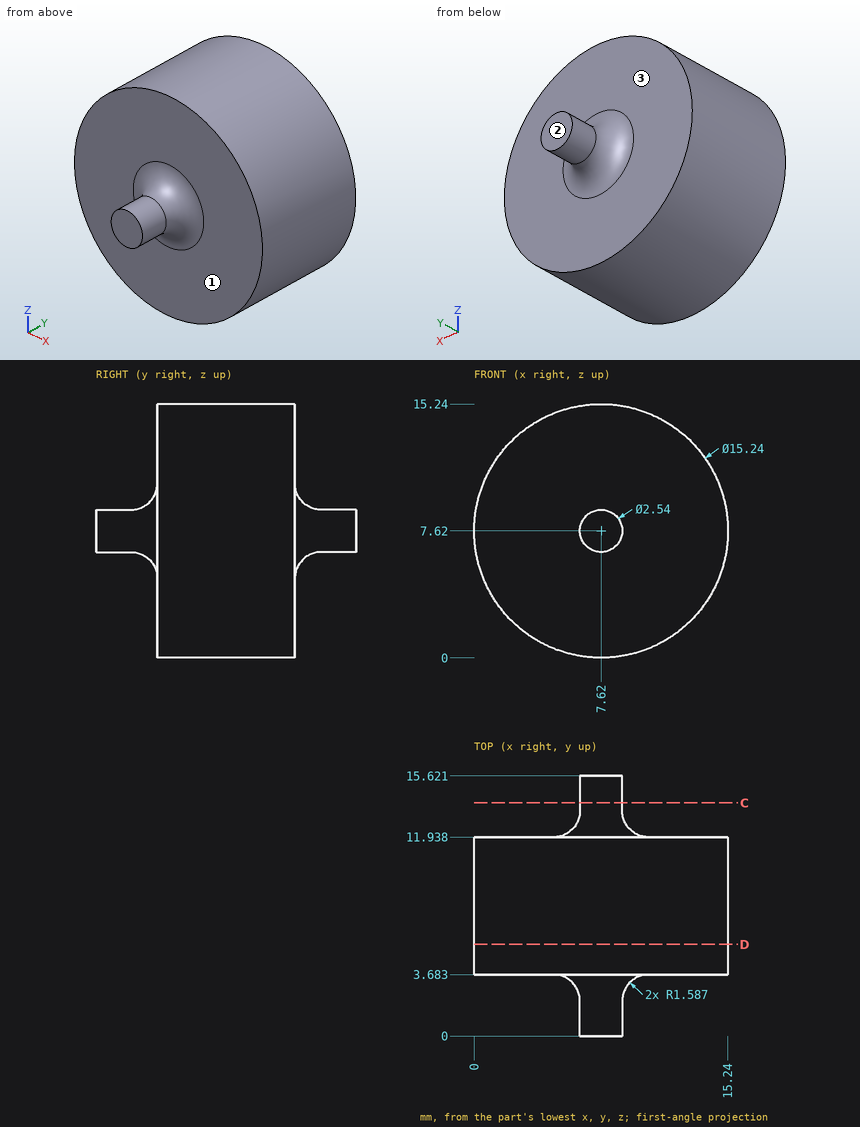
Part print with two shaded views. Sizes in mm from the minimum x, y, z corner. A direction names the side the tool comes from. Coordinates: 2 decimals unless noted, no trailing zeros. Order: outer loops, then holes, each group sorted by start corner. A loop starts at its lowest first (then second) coordinate and runs counter-clockwise, first axis right, second up.
(1) Saw through at D-D, the plane y = 5.5. Write the cut outline in (x, z).
Solution:
outline: circle Ø15.24 at (7.62, 7.62)
(2) Which spindle directions (+Z, -Z, +X, -X, +Y, -Y) get a long thin tool onto all of the face, cutting with end or side? Do the marked faces 1, 2 and 3. Say none if no direction does.
Solution:
face 1: -Y
face 2: +Z, -Z, +X, -X, +Y
face 3: +Y
(3) Drill centre lines: L1, parallel to Y at x = 14.25, z = 10; L2, parallel to Z at x = 8.75, y = 6.5 (1 decimal); L3, parallel to Z at x = 9.75, y = 7.75 (1 decimal). Where is each one in solid material? Low to high.
Solution:
L1: y = 3.68 to 11.94
L2: z = 0.1 to 15.2
L3: z = 0.3 to 14.9
(4) Saw through at C-C, the plane y = 14. Write the cut outline in (x, z).
Solution:
outline: circle Ø2.54 at (7.62, 7.62)
(5) Pin check, flat tips, straight feed: pin 1 Ø1.5 at (y, z) = (11, 11) entering from -X; pin 2 Ø3 at (x, y) = (2, 5.5) entering from +Z; pin 3 Ø6 at (x, z) = (3, 13.5) entering from -Y. Stop position of each tip, or through.
Solution:
pin 1: stops at x = 0.47
pin 2: stops at z = 14.03
pin 3: stops at y = 3.68
